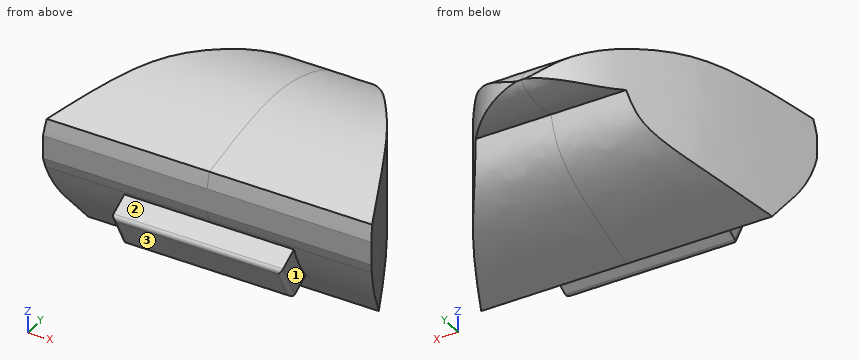
from build123d import *

# Parameters (mm, degrees)
F2_DEPTH = 7.75
F4_DEPTH = 25
F6_DEPTH = 4
F7_R     = 0.2


with BuildPart() as f2:
    # F1 (on Right) → F2 (new body, symmetric)
    with BuildSketch(Plane.YZ):
        with BuildLine():
            add(Edge.make_bspline(
                [(15.9764018067, 20.3420528816), (17.2041890595, 20.6287244677), (19.5850299616, 21.1870373625), (22.6354301881, 21.2058318383), (25.7183894409, 20.0206141081), (26.1510953936, 19.2531516386), (26.2918325878, 18.9858826508)],
                knots=[0, 0, 0, 0, 0.2959604726, 0.569686359, 0.8417277002, 1, 1, 1, 1], degree=3))
            add(Edge.make_bspline(
                [(15.907533388, 18.0637109861), (15.834929305, 18.3091583728), (15.6598763017, 19.138099244), (15.8269500679, 19.8043517568), (15.9764018067, 20.3420528816)],
                knots=[0.583290594, 0.583290594, 0.583290594, 0.583290594, 0.7059883384, 1, 1, 1, 1], degree=3))
            add(Edge.make_bspline(
                [(15.907533388, 18.0637109861), (16.3952708112, 18.2571285426), (17.5152711285, 18.7051624944), (20.8104230334, 19.6077071346), (22.5333760998, 19.128982349), (23.4615845949, 18.8083123925), (23.8998483478, 18.6566487187)],
                knots=[0, 0, 0, 0, 0.2330121711, 0.5559876221, 0.7913389708, 1, 1, 1, 1], degree=3))
            add(Edge.make_bspline(
                [(26.2918325878, 18.9858826508), (26.0522422972, 18.7461785524), (25.2037589138, 18.4974557574), (24.4436755058, 18.5382203481), (23.8998483478, 18.6566487187)],
                knots=[0, 0, 0, 0, 0.4724232135, 1, 1, 1, 1], degree=3))
        make_face()
        with BuildLine():
            add(Edge.make_bspline(
                [(15.907533388, 18.0637109861), (16.3952708112, 18.2571285426), (17.5152711285, 18.7051624944), (20.8104230334, 19.6077071346), (22.5333760998, 19.128982349), (23.4615845949, 18.8083123925), (23.8998483478, 18.6566487187)],
                knots=[0, 0, 0, 0, 0.2330121711, 0.5559876221, 0.7913389708, 1, 1, 1, 1], degree=3))
            add(Edge.make_bspline(
                [(17.872953561, 14.8083452143), (17.2104388475, 15.7501231879), (16.5534544022, 16.4581339927), (16.0339610251, 17.6363061925), (15.907533388, 18.0637109861)],
                knots=[0, 0, 0, 0, 0.3696333829, 0.583290594, 0.583290594, 0.583290594, 0.583290594], degree=3))
            add(Edge.make_bspline(
                [(23.8998483478, 18.6566487187), (23.749402857, 18.1850885688), (23.4105386945, 17.122944171), (21.2445071896, 15.8607875111), (19.0759119851, 15.1838529079), (17.872953561, 14.8083452143)],
                knots=[0, 0, 0, 0, 0.2622875414, 0.5907777464, 1, 1, 1, 1], degree=3))
        make_face()
    extrude(amount=F2_DEPTH, both=True)

    # F3 (on Top) → F4 (intersect)
    with BuildSketch(Plane.XY):
        with BuildLine():
            add(Edge.make_bspline(
                [(-7.75, 15.8), (-7.2858735782, 16.8846031645), (-5.7486243533, 20.6341718163), (-3.9473069374, 23.2912684486), (-2.0830353705, 26.1251607988), (0, 26.3124387711)],
                knots=[0, 0, 0, 0, 0.3533091933, 0.6510969403, 1, 1, 1, 1], degree=3))
            Line((-7.75, 15.8), (7.75, 15.8))
            add(Edge.make_bspline(
                [(7.75, 15.8), (7.2858735782, 16.8846031645), (5.7486243533, 20.6341718163), (3.9473069374, 23.2912684486), (2.0830353705, 26.1251607988), (0, 26.3124387711)],
                knots=[0, 0, 0, 0, 0.3533091933, 0.6510969403, 1, 1, 1, 1], degree=3))
        make_face()
    extrude(amount=F4_DEPTH, mode=Mode.INTERSECT)

    # F5 (on Right) → F6 (join, symmetric)
    with BuildSketch(Plane.YZ):
        Polygon((16.2354782637, 18.0701025299), (14.9110568744, 17.3658951857), (15.85, 15.6), (17.1744213893, 16.3042073442), align=None)
    extrude(amount=F6_DEPTH, both=True)

    # F7
    f7_edges = [f2.edges().sort_by_distance(p)[0] for p in [
        (4, 15.380528, 16.482948),
        (0, 14.911057, 17.365895),
        (-4, 15.380528, 16.482948),
        (0, 15.85, 15.6),
    ]]
    fillet(f7_edges, radius=F7_R)


solid = f2.part
For this review, take the finished solid that the model builds, in its own axes (mm). Face numbers are marked on the shaded views. Round coordinates to 2 decimals unless told otherwise and drop trailing zeros. Use a Markdown table: item, result. Add a question column.
Item 1: To check wall thickness, follow line 1 along X through (y, z) = (17, 17.25); line 2 along Z through (x, y) = (-0.75, 21); line 3 along X through (y, z) = (18.5, 15.5). State the ranges of each line that lie inside material, in increasing order.
Item 2: Mouldability with a two-part tool opening along Z and no side actions: class the marked faces 1, 2 and 3 as released by +Z, released by -Z, zero draft, split by the parting line, or undercut.
Item 3: Insertion check: pin 1 (2 mm diameter, centred on y = 16.5, z = 16.5, fed in from -X); pin 2 (3 mm diameter, centred on x = -1.5, y = 24.5, fed in from +Z); pin 3 (1.4 mm diameter, centred on y = 16, z = 16.5, fed in from +X). Each pin has a flat end and moves straight along its axis. Give the tip position at first contact, or say it passes through.
Geometry results:
| question | item | result |
|---|---|---|
| 1 | line 1 | x = -7.24 to 7.24 |
| 1 | line 2 | z = 15.88 to 21.15 |
| 1 | line 3 | x = -6.59 to 6.59 |
| 2 | face 1 | zero draft |
| 2 | face 2 | undercut |
| 2 | face 3 | released by -Z |
| 3 | pin 1 | stops at x = -7.61 |
| 3 | pin 2 | stops at z = 20.91 |
| 3 | pin 3 | stops at x = 7.55 |
